Build history of the part. All positions in model axes, mm. Face numbers are marked on the shaded views. Give positions to 0.01 mm unless a question says otherwise; leave off trailing zeros. Order: outer loops, then holes, each group sorted by start corner. A loop starts at its lowest first (then second) coordinate and runs counter-clockwise, first axis right, second up. Notation, with made-up numbers: (-12, 43.5) - (33, 43.5) arc R19 cw to (33, 65.5) - close; hole circle Ø4 at (-39, 28.25). An arc over 180 degrees is marked (long way). Write each question's results on one line, items separated by ' | '. Start each with the question number.
1) Cut at A-A on x = 0. List the corners of the cut face in (y, z), plus the area to 4 significant figures.
2) Cut at B-B on y = -14.75. List the corners of the cut face in (x, z), plus the area to 3 significant figures.
3) Drop flat-ended pins along their axis: pin 1 Ø3 at (y, z) = (-10.5, -2.5) entering from -X; pin 2 Ø4 at (y, z) = (-18.5, -2.5) entering from -X. Give the stop position or say it passes through.
4) Drill centre lines: line 1 along Z through (x, y) = (0, -17); line 2 along X through (y, z) = (-11.5, 0); line 3 along Z through (x, y) = (0.75, -17). Where is each one in solid material? Low to high. Write a range as from..to.
5) Two-plate mould, pull along X, no slides. Class the marked faces 1, 2, 3 and 4: +X half, -X half, draft (parallel to the pull), parting line (faces both ways), or undercut.
from build123d import *

# Parameters (mm, degrees)
F0_R     = 1.75
F1_DEPTH = 23
F2_R     = 1.5
F3_R     = 1
F4_DEPTH = 10


with BuildPart() as f1:
    # F0 (on Front) → F1 (new body)
    with BuildSketch(Plane.XZ):
        Polygon((-2.886751, 5), (-5.773503, 0), (-2.886751, -5), (2.886751, -5), (5.773503, 0), (2.886751, 5), align=None)
        Circle(F0_R, mode=Mode.SUBTRACT)
    extrude(amount=F1_DEPTH)

    # F2
    f2_edges = [f1.edges().sort_by_distance(p)[0] for p in [
        (2.886751, -11.5, 5),
        (-2.886751, -11.5, 5),
        (5.773503, -11.5, 0),
        (2.886751, -11.5, -5),
        (-2.886751, -11.5, -5),
        (-5.773503, -11.5, 0),
    ]]
    fillet(f2_edges, radius=F2_R)

    # F3 (on face) → F4 (cut, through all)
    with BuildSketch(Plane(origin=(4.330127, 0, -2.5), x_dir=(0, 1, 0), z_dir=(0.866025, 0, -0.5))):
        with Locations((-19.5, 0)):
            Circle(F3_R)
    extrude(amount=-F4_DEPTH, mode=Mode.SUBTRACT)


solid = f1.part
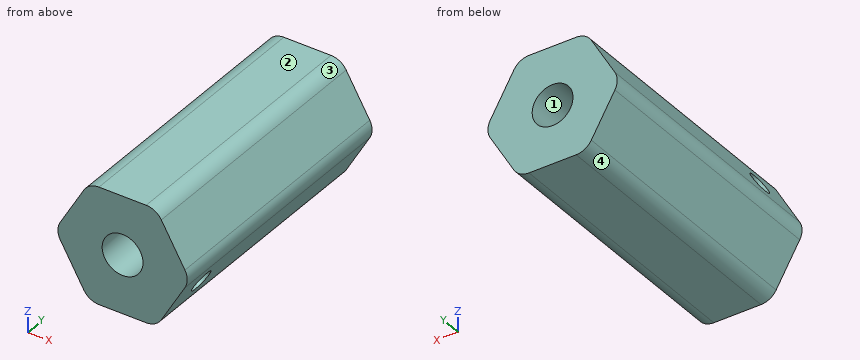
Results:
1) outline: (-23, -5) - (0, -5) - (0, -1.75) - (-23, -1.75) - close; (-23, 1.75) - (0, 1.75) - (0, 5) - (-23, 5) - close | area: 149.5 mm^2
2) outline: (-5.34, -0.75) - (-3.32, -4.25) arc R1.5 ccw to (-2.02, -5) - (2.02, -5) arc R1.5 ccw to (3.32, -4.25) - (5.34, -0.75) arc R1.5 ccw to (5.34, 0.75) - (3.32, 4.25) arc R1.5 ccw to (2.02, 5) - (-2.02, 5) arc R1.5 ccw to (-3.32, 4.25) - (-5.34, 0.75) arc R1.5 ccw to start; hole circle Ø3.5 at (0, 0) | area: 76.3 mm^2
3) pin 1: x = -5.2 | pin 2: x = -5.46
4) line 1: -5..-1.75, 1.75..5 | line 2: -5.54..-1.75, 1.75..5.54 | line 3: -5..-1.58, 1.58..5
5) face 1: undercut | face 2: draft | face 3: +X half | face 4: -X half
